```python
from build123d import *

# Parameters (mm, degrees)
SKETCH_4_R          = 1.015999997
EXTRUDE_1_DEPTH     = 2.5
SKETCH_1_R          = 1.35
SKETCH_1_R_2        = 1.3
CUT_EXTRUDE_1_DEPTH = 2.5
CUT_EXTRUDE_2_DEPTH = 2.5


with BuildPart() as part:
    # 草图4 → 凸台-拉伸1 (new body)
    with BuildSketch(Plane(origin=(0, 0, 0), x_dir=(1, 0, 0), z_dir=(0, 1, 0))):
        with BuildLine():
            Line((-42.436188428, 34.195477543), (-41.49137262, 35.131555803))
            ThreePointArc((-41.49137262, 35.131555803), (-38.877647905, 37.476008525), (-36.102115814, 39.626458957))
            ThreePointArc((-36.102115814, 39.626458957), (-33.841762455, 40.245239062), (-31.726243819, 39.236939987))
            ThreePointArc((-31.726243819, 39.236939987), (-7.620828088, 30.054645119), (16.484587642, 39.236939987))
            ThreePointArc((16.484587642, 39.236939987), (18.600106279, 40.245239062), (20.860459637, 39.626458957))
            ThreePointArc((20.860459637, 39.626458957), (23.705991726, 37.417514086), (26.38082366, 35.004680806))
            Line((26.38082366, 35.004680806), (27.30697313, 34.080620624))
            ThreePointArc((27.30697313, 34.080620624), (29.761287419, 31.369052268), (32.005630869, 28.481287726))
            ThreePointArc((32.005630869, 28.481287726), (32.159827034, 28.246667313), (32.293910707, 28))
            Line((32.293910707, 28), (39.5, 28))
            ThreePointArc((39.5, 28), (41.621320344, 27.121320344), (42.5, 25))
            Line((42.5, 25), (42.5, -25))
            ThreePointArc((42.5, -25), (41.621320344, -27.121320344), (39.5, -28))
            Line((39.5, -28), (32.293910707, -28))
            ThreePointArc((32.293910707, -28), (32.159827034, -28.246667313), (32.005630869, -28.481287726))
            ThreePointArc((32.005630869, -28.481287726), (29.775946345, -31.351575111), (27.338818851, -34.047952742))
            Line((27.338818851, -34.047952742), (26.411119263, -34.975227797))
            ThreePointArc((26.411119263, -34.975227797), (23.722187526, -37.403948618), (20.860459637, -39.626458957))
            ThreePointArc((20.860459637, -39.626458957), (18.600106279, -40.245239062), (16.484587642, -39.236939987))
            ThreePointArc((16.484587642, -39.236939987), (-7.620828088, -30.054645119), (-31.726243819, -39.236939987))
            ThreePointArc((-31.726243819, -39.236939987), (-33.841762455, -40.245239062), (-36.102115814, -39.626458957))
            ThreePointArc((-36.102115814, -39.626458957), (-39.084675426, -37.302363339), (-41.878340415, -34.754321303))
            Line((-41.878340415, -34.754321303), (-42.799522233, -33.821583024))
            ThreePointArc((-42.799522233, -33.821583024), (-45.118593637, -31.230715312), (-47.247287045, -28.481287726))
            ThreePointArc((-47.247287045, -28.481287726), (-47.86606715, -26.220934367), (-46.857768075, -24.105415731))
            ThreePointArc((-46.857768075, -24.105415731), (-44.523235736, -21.197270026), (-42.5, -18.064560362))
            Line((-42.5, -18.064560362), (-42.5, 18.064560362))
            ThreePointArc((-42.5, 18.064560362), (-44.523235736, 21.197270026), (-46.857768075, 24.105415731))
            ThreePointArc((-46.857768075, 24.105415731), (-47.86606715, 26.220934367), (-47.247287045, 28.481287726))
            ThreePointArc((-47.247287045, 28.481287726), (-44.951232672, 31.430572594), (-42.436188428, 34.195477543))
        make_face()
        with Locations((20.59934216, 36.841216125)):
            Circle(SKETCH_4_R, mode=Mode.SUBTRACT)
        with Locations((29.220388037, 28.220170249)):
            Circle(SKETCH_4_R, mode=Mode.SUBTRACT)
        with Locations((29.220388037, -28.220170249)):
            Circle(SKETCH_4_R, mode=Mode.SUBTRACT)
        with Locations((20.59934216, -36.841216125)):
            Circle(SKETCH_4_R, mode=Mode.SUBTRACT)
        with Locations((-35.840998337, -36.841216125)):
            Circle(SKETCH_4_R, mode=Mode.SUBTRACT)
        with Locations((-44.462044213, -28.220170249)):
            Circle(SKETCH_4_R, mode=Mode.SUBTRACT)
        with Locations((-35.840998337, 36.841216125)):
            Circle(SKETCH_4_R, mode=Mode.SUBTRACT)
        with Locations((-44.462044213, 28.220170249)):
            Circle(SKETCH_4_R, mode=Mode.SUBTRACT)
    extrude(amount=EXTRUDE_1_DEPTH)

    # 草图1 → 切除-拉伸1 (cut)
    with BuildSketch(Plane(origin=(0, 0, 0), x_dir=(1, 0, 0), z_dir=(0, 1, 0))):
        with Locations((19, -24.5)):
            Circle(SKETCH_1_R)
        with Locations((19, 24.5)):
            Circle(SKETCH_1_R)
        with Locations((-39, -24.5)):
            Circle(SKETCH_1_R)
        with Locations((-39, 24.5)):
            Circle(SKETCH_1_R_2)
    extrude(amount=CUT_EXTRUDE_1_DEPTH, mode=Mode.SUBTRACT)

    # 草图7 → 切除-拉伸2 (cut)
    with BuildSketch(Plane(origin=(0, 2.5, 0), x_dir=(1, 0, 0), z_dir=(0, 1, 0))):
        with BuildLine():
            Line((-1.255512377, -27.041509959), (-13.955512377, -27.041509959))
            ThreePointArc((-13.955512377, -27.041509959), (-16.649589213, -25.925586795), (-17.765512377, -23.231509959))
            Line((-17.765512377, -23.231509959), (-17.765512377, -18.151509959))
            ThreePointArc((-17.765512377, -18.151509959), (-16.649589213, -15.457433122), (-13.955512377, -14.341509959))
            Line((-13.955512377, -14.341509959), (-1.255512377, -14.341509959))
            ThreePointArc((-1.255512377, -14.341509959), (1.43856446, -15.457433122), (2.554487623, -18.151509959))
            Line((2.554487623, -18.151509959), (2.554487623, -23.231509959))
            ThreePointArc((2.554487623, -23.231509959), (1.43856446, -25.925586795), (-1.255512377, -27.041509959))
        make_face()
        with BuildLine():
            Line((6.618487623, -6.467509959), (6.618487623, 6.232490041))
            ThreePointArc((6.618487623, 6.232490041), (7.734410787, 8.926566878), (10.428487623, 10.042490041))
            Line((10.428487623, 10.042490041), (15.508487623, 10.042490041))
            ThreePointArc((15.508487623, 10.042490041), (18.20256446, 8.926566878), (19.318487623, 6.232490041))
            Line((19.318487623, 6.232490041), (19.318487623, -6.467509959))
            ThreePointArc((19.318487623, -6.467509959), (18.20256446, -9.161586795), (15.508487623, -10.277509959))
            Line((15.508487623, -10.277509959), (10.428487623, -10.277509959))
            ThreePointArc((10.428487623, -10.277509959), (7.734410787, -9.161586795), (6.618487623, -6.467509959))
        make_face()
        with BuildLine():
            Line((-1.255512377, 14.106490041), (-13.955512377, 14.106490041))
            ThreePointArc((-13.955512377, 14.106490041), (-16.649589213, 15.222413205), (-17.765512377, 17.916490041))
            Line((-17.765512377, 17.916490041), (-17.765512377, 22.996490041))
            ThreePointArc((-17.765512377, 22.996490041), (-16.649589213, 25.690566878), (-13.955512377, 26.806490041))
            Line((-13.955512377, 26.806490041), (-1.255512377, 26.806490041))
            ThreePointArc((-1.255512377, 26.806490041), (1.43856446, 25.690566878), (2.554487623, 22.996490041))
            Line((2.554487623, 22.996490041), (2.554487623, 17.916490041))
            ThreePointArc((2.554487623, 17.916490041), (1.43856446, 15.222413205), (-1.255512377, 14.106490041))
        make_face()
        with BuildLine():
            Line((-25.639512377, -10.277509959), (-30.719512377, -10.277509959))
            ThreePointArc((-30.719512377, -10.277509959), (-33.413589213, -9.161586795), (-34.529512377, -6.467509959))
            Line((-34.529512377, -6.467509959), (-34.529512377, 6.232490041))
            ThreePointArc((-34.529512377, 6.232490041), (-33.413589213, 8.926566878), (-30.719512377, 10.042490041))
            Line((-30.719512377, 10.042490041), (-25.639512377, 10.042490041))
            ThreePointArc((-25.639512377, 10.042490041), (-22.94543554, 8.926566878), (-21.829512377, 6.232490041))
            Line((-21.829512377, 6.232490041), (-21.829512377, -6.467509959))
            ThreePointArc((-21.829512377, -6.467509959), (-22.94543554, -9.161586795), (-25.639512377, -10.277509959))
        make_face()
    extrude(amount=-CUT_EXTRUDE_2_DEPTH, mode=Mode.SUBTRACT)


solid = part.part
```
The listing builds one solid part. Answer for the finished solid, in the listing's coordinates (mm). A direction names the side the tool comes from. Coordinates: 2 decimals unless noted, no trailing zeros. Loops run counter-clockwise (first coordinate to the right, second up) from the corner with the lowest first, then second, coordinate; pieces in that order, holes last. Notation, with made-up numbers: (25.25, 78.5) - (39.25, 78.5) arc R11 ccw to (39.25, 91.5) - close; hole circle Ø1 at (16, 88.25). An arc over 180 degrees is marked (long way). Write item = value, one per line.
1) Section D-D (z = -32.5) is taken. Determine the outline of the cut face in (x, y), plus the area to 3 significant figures.
Responses:
outline = (-44.02, 0) - (-20.71, 0) - (-20.71, 2.5) - (-44.02, 2.5) - close; (5.46, 0) - (28.78, 0) - (28.78, 2.5) - (5.46, 2.5) - close
area = 117 mm^2
2) Each of these flat-tipped pins is pushed along its axis until it touches: P1, Ø0.8, axis at y = 2, z = 3, coming from the -X side; P2, Ø0.8, axis at x = 35.5, y = 1, coming from the -Z side; P3, Ø1, axis at x = -24.5, y = 0.5, coming from the +Z side. Where does it stop, or does it pass through?
Responses:
P1 = -42.5
P2 = -28
P3 = 34.49
3) Find the intervals of material crossed by line 1 along X through (y, z) = (2.25, 3.5); line 2 along Z through (x, y) = (28.5, 0.5); line 3 along Z through (x, y) = (-14, 2.25), in increasing order.
Responses:
line_1 = -42.5 to -34.53, -21.83 to 6.62, 19.32 to 42.5
line_2 = -32.81 to -28.94, -27.5 to 27.5, 28.94 to 32.81
line_3 = -30.62 to -26.81, -14.11 to 14.34, 27.04 to 30.62
4) Section B-B (x = -7) is taken. Determine the outline of the cut face in (y, z), plus the area to 3 significant figures.
Responses:
outline = (0, -30.06) - (2.5, -30.06) - (2.5, -26.81) - (0, -26.81) - close; (0, -14.11) - (2.5, -14.11) - (2.5, 14.34) - (0, 14.34) - close; (0, 27.04) - (2.5, 27.04) - (2.5, 30.06) - (0, 30.06) - close
area = 86.8 mm^2
5) Section C-C (z = 22) is taken. Determine the outline of the cut face in (x, y), plus the area to 3 significant figures.
Responses:
outline = (-45.12, 0) - (-17.77, 0) - (-17.77, 2.5) - (-45.12, 2.5) - close; (2.55, 0) - (42.5, 0) - (42.5, 2.5) - (2.55, 2.5) - close
area = 168 mm^2
6) Determine the mould class of faces 1 (the face through (2.554, 1, 21)), 2 (the face through (23.67, 1.23, -37.45)), 3 (the face through (36, 1, 28)) for opening direction Z: pulls with the +Z half, pulls with the -Z half, needs draft (parallel to the pull), parting line crosses it, or undercut.
Responses:
face_1 = undercut
face_2 = pulls with the -Z half
face_3 = pulls with the +Z half
7) Section A-A (z = -5) is taken. Determine the outline of the cut face in (x, y), plus the area to 3 significant figures.
Responses:
outline = (-42.5, 0) - (-34.53, 0) - (-34.53, 2.5) - (-42.5, 2.5) - close; (-21.83, 0) - (6.62, 0) - (6.62, 2.5) - (-21.83, 2.5) - close; (19.32, 0) - (42.5, 0) - (42.5, 2.5) - (19.32, 2.5) - close
area = 149 mm^2
8) Which of the six approach directions +Z, -Z, +X, -X, +Y, -Y give full straight-line access (tool end or side, diameter ignored) to faces 4 (the face through (19.318, 1, 0)), 5 (the face through (-44.49, 1.23, -21.15)), 6 (the face through (-38.92, 1.23, -37.44))?
Responses:
face_4 = +Y, -Y
face_5 = -X, +Y, -Y
face_6 = -Z, -X, +Y, -Y
